```python
from build123d import *

# Parameters (mm, degrees)
SKETCH_1_W      = 2
SKETCH_1_H      = 6
EXTRUDE_1_DEPTH = 2


with BuildPart() as part:
    # 草图1 → 凸台-拉伸1 (new body)
    with BuildSketch(Plane.XY):
        Polygon((529.48584496, 31.739769875), (4.48584496, 31.739769875), (4.48584496, 21.739769875), (6.48584496, 21.739769875), (6.48584496, 15.739769875), (4.48584496, 15.739769875), (4.48584496, 5.770075294), (529.48584496, 13.938813064), (529.48584496, 19.739769875), (527.48584496, 19.739769875), (527.48584496, 25.739769875), (529.48584496, 25.739769875), align=None)
        with Locations((140.48584496, 19.739769875)):
            Rectangle(SKETCH_1_W, SKETCH_1_H, mode=Mode.SUBTRACT)
        with Locations((280.48584496, 20.739769875)):
            Rectangle(SKETCH_1_W, SKETCH_1_H, mode=Mode.SUBTRACT)
        with Locations((410.48584496, 21.739769875)):
            Rectangle(SKETCH_1_W, SKETCH_1_H, mode=Mode.SUBTRACT)
        with BuildLine():
            Line((13.48584496, 22.739769875), (13.48584496, 14.973438176))
            ThreePointArc((13.48584496, 14.973438176), (14.679505875, 12.123094173), (17.54807543, 10.973922284))
            Line((17.54807543, 10.973922284), (47.04807543, 11.43292755))
            ThreePointArc((47.04807543, 11.43292755), (49.836188964, 12.626104356), (50.98584496, 15.432443441))
            Line((50.98584496, 15.432443441), (50.98584496, 22.739769875))
            ThreePointArc((50.98584496, 22.739769875), (49.814272085, 25.568196999), (46.98584496, 26.739769875))
            Line((46.98584496, 26.739769875), (17.48584496, 26.739769875))
            ThreePointArc((17.48584496, 26.739769875), (14.657417835, 25.568196999), (13.48584496, 22.739769875))
        make_face(mode=Mode.SUBTRACT)
        with BuildLine():
            Line((55.98584496, 22.739769875), (55.98584496, 15.634716948))
            ThreePointArc((55.98584496, 15.634716948), (57.179505875, 12.784372944), (60.04807543, 11.635201056))
            Line((60.04807543, 11.635201056), (86.04807543, 12.03974807))
            ThreePointArc((86.04807543, 12.03974807), (88.836188964, 13.232924876), (89.98584496, 16.039263961))
            Line((89.98584496, 16.039263961), (89.98584496, 22.739769875))
            ThreePointArc((89.98584496, 22.739769875), (88.814272085, 25.568196999), (85.98584496, 26.739769875))
            Line((85.98584496, 26.739769875), (59.98584496, 26.739769875))
            ThreePointArc((59.98584496, 26.739769875), (57.157417835, 25.568196999), (55.98584496, 22.739769875))
        make_face(mode=Mode.SUBTRACT)
        with BuildLine():
            Line((94.98584496, 22.739769875), (94.98584496, 16.241537468))
            ThreePointArc((94.98584496, 16.241537468), (96.179505875, 13.391193464), (99.04807543, 12.242021576))
            Line((99.04807543, 12.242021576), (128.54807543, 12.701026841))
            ThreePointArc((128.54807543, 12.701026841), (131.336188964, 13.894203648), (132.48584496, 16.700542733))
            Line((132.48584496, 16.700542733), (132.48584496, 22.739769875))
            ThreePointArc((132.48584496, 22.739769875), (131.314272085, 25.568196999), (128.48584496, 26.739769875))
            Line((128.48584496, 26.739769875), (98.98584496, 26.739769875))
            ThreePointArc((98.98584496, 26.739769875), (96.157417835, 25.568196999), (94.98584496, 22.739769875))
        make_face(mode=Mode.SUBTRACT)
        with BuildLine():
            Line((148.48584496, 22.739769875), (148.48584496, 17.073970745))
            ThreePointArc((148.48584496, 17.073970745), (149.679505875, 14.223626742), (152.54807543, 13.074454854))
            Line((152.54807543, 13.074454854), (183.04807543, 13.549019619))
            ThreePointArc((183.04807543, 13.549019619), (185.836188964, 14.742196426), (186.98584496, 17.548535511))
            Line((186.98584496, 17.548535511), (186.98584496, 22.739769875))
            ThreePointArc((186.98584496, 22.739769875), (185.814272085, 25.568196999), (182.98584496, 26.739769875))
            Line((182.98584496, 26.739769875), (152.48584496, 26.739769875))
            ThreePointArc((152.48584496, 26.739769875), (149.657417835, 25.568196999), (148.48584496, 22.739769875))
        make_face(mode=Mode.SUBTRACT)
        with BuildLine():
            Line((191.98584496, 22.739769875), (191.98584496, 17.750809018))
            ThreePointArc((191.98584496, 17.750809018), (193.179505875, 14.900465014), (196.04807543, 13.751293126))
            Line((196.04807543, 13.751293126), (225.04807543, 14.202518641))
            ThreePointArc((225.04807543, 14.202518641), (227.836188964, 15.395695448), (228.98584496, 18.202034533))
            Line((228.98584496, 18.202034533), (228.98584496, 22.739769875))
            ThreePointArc((228.98584496, 22.739769875), (227.814272085, 25.568196999), (224.98584496, 26.739769875))
            Line((224.98584496, 26.739769875), (195.98584496, 26.739769875))
            ThreePointArc((195.98584496, 26.739769875), (193.157417835, 25.568196999), (191.98584496, 22.739769875))
        make_face(mode=Mode.SUBTRACT)
        with BuildLine():
            Line((233.98584496, 22.739769875), (233.98584496, 18.404308039))
            ThreePointArc((233.98584496, 18.404308039), (235.179505875, 15.553964036), (238.04807543, 14.404792148))
            Line((238.04807543, 14.404792148), (268.54807543, 14.879356913))
            ThreePointArc((268.54807543, 14.879356913), (271.336188964, 16.07253372), (272.48584496, 18.878872805))
            Line((272.48584496, 18.878872805), (272.48584496, 22.739769875))
            ThreePointArc((272.48584496, 22.739769875), (271.314272085, 25.568196999), (268.48584496, 26.739769875))
            Line((268.48584496, 26.739769875), (237.98584496, 26.739769875))
            ThreePointArc((237.98584496, 26.739769875), (235.157417835, 25.568196999), (233.98584496, 22.739769875))
        make_face(mode=Mode.SUBTRACT)
        with BuildLine():
            Line((288.48584496, 22.739769875), (288.48584496, 19.252300817))
            ThreePointArc((288.48584496, 19.252300817), (289.679505875, 16.401956814), (292.54807543, 15.252784926))
            Line((292.54807543, 15.252784926), (320.04807543, 15.68067119))
            ThreePointArc((320.04807543, 15.68067119), (322.836188964, 16.873847996), (323.98584496, 19.680187081))
            Line((323.98584496, 19.680187081), (323.98584496, 22.739769875))
            ThreePointArc((323.98584496, 22.739769875), (322.814272085, 25.568196999), (319.98584496, 26.739769875))
            Line((319.98584496, 26.739769875), (292.48584496, 26.739769875))
            ThreePointArc((292.48584496, 26.739769875), (289.657417835, 25.568196999), (288.48584496, 22.739769875))
        make_face(mode=Mode.SUBTRACT)
        with BuildLine():
            Line((328.98584496, 22.739769875), (328.98584496, 19.882460588))
            ThreePointArc((328.98584496, 19.882460588), (330.179505875, 17.032116584), (333.04807543, 15.882944696))
            Line((333.04807543, 15.882944696), (358.04807543, 16.271932209))
            ThreePointArc((358.04807543, 16.271932209), (360.836188964, 17.465109016), (361.98584496, 20.271448101))
            Line((361.98584496, 20.271448101), (361.98584496, 22.739769875))
            ThreePointArc((361.98584496, 22.739769875), (360.814272085, 25.568196999), (357.98584496, 26.739769875))
            Line((357.98584496, 26.739769875), (332.98584496, 26.739769875))
            ThreePointArc((332.98584496, 26.739769875), (330.157417835, 25.568196999), (328.98584496, 22.739769875))
        make_face(mode=Mode.SUBTRACT)
        with BuildLine():
            Line((366.98584496, 22.739769875), (366.98584496, 20.473721608))
            ThreePointArc((366.98584496, 20.473721608), (368.179505875, 17.623377604), (371.04807543, 16.474205716))
            Line((371.04807543, 16.474205716), (398.54807543, 16.90209198))
            ThreePointArc((398.54807543, 16.90209198), (401.336188964, 18.095268787), (402.48584496, 20.901607872))
            Line((402.48584496, 20.901607872), (402.48584496, 22.739769875))
            ThreePointArc((402.48584496, 22.739769875), (401.314272085, 25.568196999), (398.48584496, 26.739769875))
            Line((398.48584496, 26.739769875), (370.98584496, 26.739769875))
            ThreePointArc((370.98584496, 26.739769875), (368.157417835, 25.568196999), (366.98584496, 22.739769875))
        make_face(mode=Mode.SUBTRACT)
        with BuildLine():
            Line((418.48584496, 22.739769875), (418.48584496, 21.275035884))
            ThreePointArc((418.48584496, 21.275035884), (419.679505875, 18.42469188), (422.54807543, 17.275519992))
            Line((422.54807543, 17.275519992), (447.04807543, 17.656727755))
            ThreePointArc((447.04807543, 17.656727755), (449.836188964, 18.849904561), (450.98584496, 21.656243647))
            Line((450.98584496, 21.656243647), (450.98584496, 22.739769875))
            ThreePointArc((450.98584496, 22.739769875), (449.814272085, 25.568196999), (446.98584496, 26.739769875))
            Line((446.98584496, 26.739769875), (422.48584496, 26.739769875))
            ThreePointArc((422.48584496, 26.739769875), (419.657417835, 25.568196999), (418.48584496, 22.739769875))
        make_face(mode=Mode.SUBTRACT)
        with BuildLine():
            Line((455.98584496, 22.739769875), (455.98584496, 21.858517153))
            ThreePointArc((455.98584496, 21.858517153), (457.179505875, 19.00817315), (460.04807543, 17.859001262))
            Line((460.04807543, 17.859001262), (481.04807543, 18.185750772))
            ThreePointArc((481.04807543, 18.185750772), (483.836188964, 19.378927579), (484.98584496, 22.185266664))
            Line((484.98584496, 22.185266664), (484.98584496, 22.739769875))
            ThreePointArc((484.98584496, 22.739769875), (483.814272085, 25.568196999), (480.98584496, 26.739769875))
            Line((480.98584496, 26.739769875), (459.98584496, 26.739769875))
            ThreePointArc((459.98584496, 26.739769875), (457.157417835, 25.568196999), (455.98584496, 22.739769875))
        make_face(mode=Mode.SUBTRACT)
        with BuildLine():
            Line((489.98584496, 22.739769875), (489.98584496, 22.387540171))
            ThreePointArc((489.98584496, 22.387540171), (491.179505875, 19.537196167), (494.04807543, 18.388024279))
            Line((494.04807543, 18.388024279), (519.532517812, 18.784549473))
            ThreePointArc((519.532517812, 18.784549473), (521.623602963, 19.679432078), (522.48584496, 21.784186392))
            Line((522.48584496, 21.784186392), (522.48584496, 23.739769875))
            ThreePointArc((522.48584496, 23.739769875), (521.607165304, 25.861090218), (519.48584496, 26.739769875))
            Line((519.48584496, 26.739769875), (493.98584496, 26.739769875))
            ThreePointArc((493.98584496, 26.739769875), (491.157417835, 25.568196999), (489.98584496, 22.739769875))
        make_face(mode=Mode.SUBTRACT)
    extrude(amount=EXTRUDE_1_DEPTH)


solid = part.part
```
Work out the finished part from the listing and answer in its coordinate system (mm). Coordinates: 2 decimals unless noted, no trailing zeros. Loops run counter-clockwise (first coordinate to the right, second up) from the corner with the lowest first, then second, coordinate; pieces in that order, holes last. Notation, with made-up numbers: (44.5, -34.75) -> (63.5, -34.75) arc R13 ccw to (63.5, -10.75) -> close; hole circle Ø9 at (89.5, 84). An arc over 180 degrees is marked (long way). Answer as CSV lines item,"result".
Q1. Find the intervals of material crossed by probe 1 along Y at (x, z) = (438.5, 1.5); probe 2 along Y at (x, z) = (206, 1.65); probe 3 along Y at (x, z) = (52, 1.7), in increasing order.
Findings:
probe 1,"y = 12.52 to 17.52, 26.74 to 31.74"
probe 2,"y = 8.91 to 13.91, 26.74 to 31.74"
probe 3,"y = 6.51 to 31.74"
Q2. The part is cut by section B-B on z = 1.35. State how many separate pieces and enclosed holes the cut face has, and give its area (3 significant figures).
Findings:
separate pieces,"1"
enclosed holes,"15"
area,"6,580 mm²"
Q3. The part is cut by section A-A on x = 172.5. Write down the section's boundary in (y, z), and give its area (3 significant figures).
Findings:
outline,"(8.38, 0) -> (13.38, 0) -> (13.38, 2) -> (8.38, 2) -> close; (26.74, 0) -> (31.74, 0) -> (31.74, 2) -> (26.74, 2) -> close"
area,"20.0 mm²"
Q4. Each of these flat-tipped pins is pushed along its axis until it touches: pin 1 (1 mm diameter, centred on y = 20.5, z = 1, fed in from -X); pin 2 (1 mm diameter, centred on x = 341, z = 1, fed in from -Y); pin 3 (0.6 mm diameter, centred on x = 35.5, z = 1.5, fed in from -Y); pin 4 (0.6 mm diameter, centred on y = 21.5, z = 1, fed in from -X). Where does it stop, or does it pass through?
Findings:
pin 1,"stops at x = 6.49"
pin 2,"stops at y = 11"
pin 3,"stops at y = 6.25"
pin 4,"stops at x = 4.49"
